Geometry: final body of the model. Coordinates: model frame, mm. Face numbers are marked on the shaded views. A direction names the side the tool comes from. Coordinates: 2 decimals unless noted, no trailing zeros. Write each loop counter-clockwise with the first axis right and the second up, starting at its lowest first coordinate (ties: lowest second). Pieces come first, ordered by that corner, then holes. Notation, with made-up numbers: (39, 51) - (54, 51) arc R16 cw to (54, 76) - close; hole circle Ø1 at (36, 17). An arc over 180 degrees is marked (long way). Answer as a JSON object with one key per item and string values. Group by question number.
Item 1: Line query: line 1 along Y through (x, z) = (-16.5, -11); line 2 along X through (y, z) = (113, 22.5). Output: solid intervals per line, ascending. Write a range as from..to.
Item 2: Set-up query: the marked faces 1, 2, 3, 4 and 5. Return all of +Z, -Z, +X, -X, +Y, -Y with unobstructed straight access to the full face (end or side cutting, diameter ignored); none if empty.
Item 3: Section A-A on x = -6. Return loops of the section in (y, z), and give its area (3 significant figures).
Item 4: Section C-C on y = -17. Return loops of the section in (x, z).
Item 5: First-contact query: pin 1 Ø15 at (y, z) = (-30, -9) entering from +X; pin 2 Ø6 at (x, z) = (3, 16) entering from -Y; pin 3 Ø3 at (x, z) = (10, -10.5) entering from +Y. Flat tips, straight axial feed; report the tip coordinate or a pass-through.
Item 6: Section B-B on z = 22. Return loops of the section in (x, y), and give its area (3 significant figures).
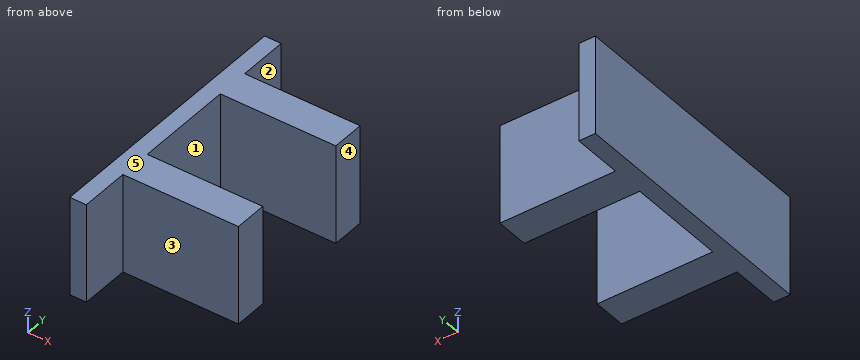
```python
from build123d import *

# Parameters (mm, degrees)
F1_DEPTH = 10
F2_W     = 10
F2_H     = 60
F3_DEPTH = 30


with BuildPart() as f1:
    # F0 (on Front) → F1 (new body)
    with BuildSketch(Plane.XZ):
        Polygon((40, 0), (10, 30), (-40, 30), (-40, -30), (40, -30), align=None)
    extrude(amount=F1_DEPTH)

    # F2 (on face) → F3 (join)
    with BuildSketch(Plane.XZ.offset(10)):
        with Locations((-35, 0)):
            Rectangle(F2_W, F2_H)
    extrude(amount=F3_DEPTH)

    # F4: F1 across plane


with BuildPart() as f1_1:
    add(f1.part)
    add(f1.part.mirror(Plane.XY))

    # F5: F1 across face


with BuildPart() as f1_2:
    add(f1_1.part)
    add(f1_1.part.mirror(Plane(origin=(0, 0, 0), x_dir=(-1, 0, 0), z_dir=(0, 1, 0))))

    # F6: F1 across face


with BuildPart() as f1_3:
    add(f1_2.part)
    add(f1_2.part.mirror(Plane(origin=(-35, 40, 0), x_dir=(-1, 0, 0), z_dir=(0, 1, 0))))


solid = f1_3.part
```
Checks:
{
 "1": {"line 1": "-10..10, 70..90", "line 2": "-40..-30"},
 "2": {"face 1": "+Z, -Z, +X", "face 2": "+Z, -Z, +X, +Y", "face 3": "+Z, -Z, +X, -Y", "face 4": "+Z, -Z, +X, +Y, -Y", "face 5": "+Z, +X, -X, +Y, -Y"},
 "3": {"outline": "(-10, -30) - (10, -30) - (10, 30) - (-10, 30) - close; (70, -30) - (90, -30) - (90, 30) - (70, 30) - close", "area": "2,400 mm^2"},
 "4": {"outline": "(-40, -30) - (-30, -30) - (-30, 30) - (-40, 30) - close"},
 "5": {"pin 1": "x = -30", "pin 2": "y = -10", "pin 3": "y = 90"},
 "6": {"outline": "(-40, -40) - (-30, -40) - (-30, -10) - (40, -10) - (40, 10) - (-30, 10) - (-30, 70) - (40, 70) - (40, 90) - (-30, 90) - (-30, 120) - (-40, 120) - close", "area": "4,400 mm^2"}
}
